from build123d import *

# Parameters (mm, degrees)
BOSS_EXTRUDE1_DEPTH = 35
SKETCH2_W           = 6.5
SKETCH2_H           = 4.4
CUT_EXTRUDE1_DEPTH  = 3
SKETCH3_W           = 3
SKETCH3_H           = 3
BOSS_EXTRUDE2_DEPTH = 5
SKETCH4_W           = 0.2
SKETCH4_H           = 0.2
CUT_EXTRUDE2_DEPTH  = 73.994691588


with BuildPart() as part:
    # Sketch1 → Boss-Extrude1 (new, symmetric)
    with BuildSketch(Plane.XY):
        with BuildLine():
            Line((-28, 9.65), (28, 9.65))
            ThreePointArc((28, 9.65), (30.121320344, 8.771320344), (31, 6.65))
            Line((31, 6.65), (31, -6.65))
            ThreePointArc((31, -6.65), (30.121320344, -8.771320344), (28, -9.65))
            Line((28, -9.65), (-28, -9.65))
            ThreePointArc((-28, -9.65), (-30.121320344, -8.771320344), (-31, -6.65))
            Line((-31, -6.65), (-31, 6.65))
            ThreePointArc((-31, 6.65), (-30.121320344, 8.771320344), (-28, 9.65))
        make_face()
    extrude(amount=BOSS_EXTRUDE1_DEPTH, both=True)

    # Sketch2 → Cut-Extrude1 (cut)
    with BuildSketch(Plane(origin=(0, 9.65, 0), x_dir=(1, 0, 0), z_dir=(0, 1, 0))):
        with Locations((-18.75, -28.55)):
            Rectangle(SKETCH2_W, SKETCH2_H)
    extrude(amount=-CUT_EXTRUDE1_DEPTH, mode=Mode.SUBTRACT)

    # Sketch3 → Boss-Extrude2 (add)
    with BuildSketch(Plane(origin=(0, 6.65, 0), x_dir=(1, 0, 0), z_dir=(0, 1, 0))):
        with Locations((-20.4, -28.55)):
            Rectangle(SKETCH3_W, SKETCH3_H)
    extrude(amount=BOSS_EXTRUDE2_DEPTH)

    # Sketch4 → Cut-Extrude2 (cut, through all)
    with BuildSketch(Plane.XY.offset(30.05)):
        with Locations((-21.602270094, 11.55)):
            Rectangle(SKETCH4_W, SKETCH4_H)
        with Locations((-21.202270094, 11.55)):
            Rectangle(SKETCH4_W, SKETCH4_H)
        with Locations((-20.802270094, 11.55)):
            Rectangle(SKETCH4_W, SKETCH4_H)
        with Locations((-20.402270094, 11.55)):
            Rectangle(SKETCH4_W, SKETCH4_H)
        with Locations((-20.002270094, 11.55)):
            Rectangle(SKETCH4_W, SKETCH4_H)
        with Locations((-19.602270094, 11.55)):
            Rectangle(SKETCH4_W, SKETCH4_H)
        with Locations((-19.202270094, 11.55)):
            Rectangle(SKETCH4_W, SKETCH4_H)
    extrude(amount=-CUT_EXTRUDE2_DEPTH, mode=Mode.SUBTRACT)


solid = part.part
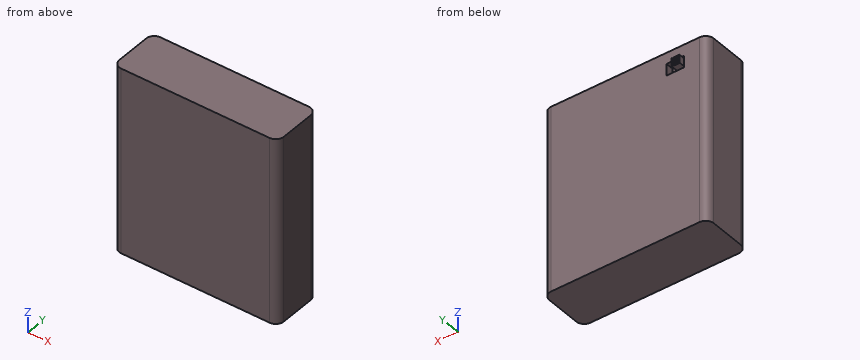
Model file for the job. Use its own axes, mm. Give positions to 0.01 mm unless a question says otherwise; leave off trailing zeros. Order: outer loops, then holes, each group sorted by start corner. A loop starts at its lowest first (then second) coordinate and runs counter-clockwise, first axis right, second up. Notation, with made-up numbers: M 80.5,26 L 104.5,26 A30 ccw 104.5,65 Z; hole C -19,81.5 d6. An arc over 180 degrees is marked long. Put each result on its own line as item: value. Start each with the question number.
(1) Band-saw the part on B-B on z = -28.5. Give the cut face in (x, y), then the cut area to 3 significant figures.
(2) Band-saw the part on A-A on y = 8.25. Give the cut face in (x, z).
(3) Pin check, flat tips, straight feed: pin 1 Ø2.5 at (x, y) = (-20, 10.5) entering from -Z; pin 2 Ø0.9 at (y, z) = (8.5, 29.5) entering from -X; pin 3 Ø0.9 at (y, z) = (8.5, 27.5) entering from +X; pin 4 Ø4 at (x, z) = (10.5, -8) entering from +Y. Stop position of each tip, or through.
(4) Band-saw the part on C-C on x = -18. Give the cut face in (y, z).
(5) Drill centre lines: L1, parallel to Y at x = -19.5, z = -24.5; L2, parallel to X at y = 9, z = 17.5. Where is each one in solid material? Low to high. Write a range as [from, to].
(6) Band-saw the part on D-D on x = 12.5. Give the cut face in (y, z).
Results below:
1. outline: M -31,-6.65 A3 ccw -28,-9.65 L 28,-9.65 A3 ccw 31,-6.65 L 31,6.65 A3 ccw 28,9.65 L -28,9.65 A3 ccw -31,6.65 Z
1. area: 1,190 mm2
2. outline: M -30.54,-35 L 30.54,-35 L 30.54,35 L -30.54,35 Z; M -21.9,27.05 L -18.9,27.05 L -18.9,30.05 L -21.9,30.05 Z; hole M -22,26.35 L -15.5,26.35 L -15.5,30.75 L -22,30.75 Z
3. pin 1: stops at z = -35
3. pin 2: stops at x = -30.65
3. pin 3: stops at x = 30.65
3. pin 4: stops at y = 9.65
4. outline: M -9.65,-35 L 9.65,-35 L 9.65,26.35 L 6.65,26.35 L 6.65,30.75 L 9.65,30.75 L 9.65,35 L -9.65,35 Z
5. L1: y = [-9.65, 9.65]
5. L2: x = [-29.86, 29.86]
6. outline: M -9.65,-35 L 9.65,-35 L 9.65,35 L -9.65,35 Z
